Geometry: final body of the model. Coordinates: model frame, mm. Face numbers are marked on the shaded views. A direction names the side the tool comes from. Give positions to 0.01 mm unless a question says otherwise; leave off trailing zeros. Order: outer loops, then holes, each group sorted by start corner. A loop starts at its lowest first (then second) coordinate and runs counter-clockwise, first axis right, second up. Notation, with made-up numbers: (17.25, 14.5) - (47.25, 14.5) arc R28 ccw to (47.25, 48.5) - close; hole circle Ø10 at (4.25, 48). An arc over 180 degrees is marked (long way). One line per item, written item: value.
```python
from build123d import *

# Parameters (mm, degrees)
SKETCH3_W           = 50.6
SKETCH3_H           = 54.3
SKETCH3_W_2         = 44.9
SKETCH3_H_2         = 48.6
BOSS_EXTRUDE1_DEPTH = 32
FILLET1_R           = 2
FILLET2_R           = 1


with BuildPart() as part:
    # Sketch3 → Boss-Extrude1 (new body)
    with BuildSketch(Plane(origin=(0, 0, 0), x_dir=(1, 0, 0), z_dir=(0, 1, 0))):
        Rectangle(SKETCH3_W, SKETCH3_H)
        Rectangle(SKETCH3_W_2, SKETCH3_H_2, mode=Mode.SUBTRACT)
    extrude(amount=BOSS_EXTRUDE1_DEPTH)

    # Fillet1
    fillet1_edges = [part.edges().sort_by_distance(p)[0] for p in [
        (25.3, 16, 27.15),
        (-25.3, 16, 27.15),
        (-25.3, 16, -27.15),
        (25.3, 16, -27.15),
    ]]
    fillet(fillet1_edges, radius=FILLET1_R)

    # Fillet2
    fillet2_edges = [part.edges().sort_by_distance(p)[0] for p in [
        (22.45, 16, 24.3),
        (22.45, 16, -24.3),
        (-22.45, 16, -24.3),
        (-22.45, 16, 24.3),
    ]]
    fillet(fillet2_edges, radius=FILLET2_R)


solid = part.part
```
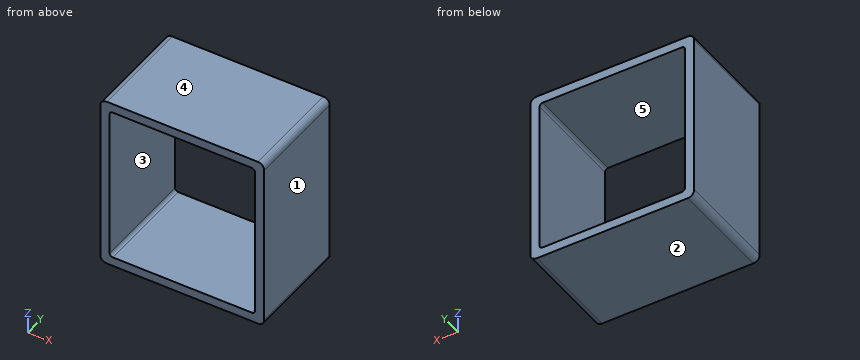
1) Set-up query: the marked faces 4 and 5. Return all of +Z, -Z, +X, -X, +Y, -Y with unobstructed straight access to the full face (end or side cutting, diameter ignored); none if empty.
Answers below:
face 4: +Z, +X, -X, +Y, -Y
face 5: +Y, -Y
2) Mould query, pull axis Z, two halves, no side actions, for the marked faces 1, 2 and 3. Classes: released by +Z, released by -Z, zero draft, split by the parting line, or undercut.
Answers below:
face 1: zero draft
face 2: released by -Z
face 3: undercut
3) Section A-A, the plane x = 14.5. Return loops of the section in (y, z).
Answers below:
outline: (0, -27.15) - (32, -27.15) - (32, -24.3) - (0, -24.3) - close; (0, 24.3) - (32, 24.3) - (32, 27.15) - (0, 27.15) - close
4) Section B-B, the plane z = 14. Return loops of the section in (x, y), then the cut area to 3 significant figures.
Answers below:
outline: (-25.3, 0) - (-22.45, 0) - (-22.45, 32) - (-25.3, 32) - close; (22.45, 0) - (25.3, 0) - (25.3, 32) - (22.45, 32) - close
area: 182 mm^2
5) Section C-C, the plane y = 24. Return loops of the section in (x, z).
Answers below:
outline: (-25.3, -25.15) arc R2 ccw to (-23.3, -27.15) - (23.3, -27.15) arc R2 ccw to (25.3, -25.15) - (25.3, 25.15) arc R2 ccw to (23.3, 27.15) - (-23.3, 27.15) arc R2 ccw to (-25.3, 25.15) - close; hole (-22.45, -23.3) arc R1 ccw to (-21.45, -24.3) - (21.45, -24.3) arc R1 ccw to (22.45, -23.3) - (22.45, 23.3) arc R1 ccw to (21.45, 24.3) - (-21.45, 24.3) arc R1 ccw to (-22.45, 23.3) - close
6) Material intervals for line 1 along Z through (x, y) = (16, 28); line 2 along X through (y, z) = (25.5, 10); line 3 along X through (y, z) = (19, 24), sorted ascending.
Answers below:
line 1: -27.15 to -24.3, 24.3 to 27.15
line 2: -25.3 to -22.45, 22.45 to 25.3
line 3: -25.3 to -22.16, 22.16 to 25.3
